```python
from build123d import *

# Parameters (mm, degrees)
BOSS_EXTRUDE1_DEPTH = 12.05
SKETCH2_R           = 1.25
BOSS_EXTRUDE2_DEPTH = 2.5
BOSS_EXTRUDE3_DEPTH = 4.4
SKETCH4_R           = 0.5
BOSS_EXTRUDE4_DEPTH = 3.7
CHAMFER1_SIZE       = 0.1


with BuildPart() as part:
    # Sketch1 → Boss-Extrude1 (new body, symmetric)
    with BuildSketch(Plane.XY):
        with BuildLine():
            Line((-5.6, -11.5), (5.6, -11.5))
            ThreePointArc((5.6, -11.5), (5.953553391, -11.353553391), (6.1, -11))
            Line((6.1, -11), (6.1, 11))
            ThreePointArc((6.1, 11), (5.953553391, 11.353553391), (5.6, 11.5))
            Line((5.6, 11.5), (-5.6, 11.5))
            ThreePointArc((-5.6, 11.5), (-5.953553391, 11.353553391), (-6.1, 11))
            Line((-6.1, 11), (-6.1, -11))
            ThreePointArc((-6.1, -11), (-5.953553391, -11.353553391), (-5.6, -11.5))
        make_face()
    extrude(amount=BOSS_EXTRUDE1_DEPTH, both=True)

    # Sketch2 → Boss-Extrude2 (add)
    with BuildSketch(Plane.XY.offset(-7.75)):
        with BuildLine():
            Line((6.1, 11), (6.1, 15.65))
            ThreePointArc((6.1, 15.65), (5.953553391, 16.003553391), (5.6, 16.15))
            Line((5.6, 16.15), (-5.6, 16.15))
            ThreePointArc((-5.6, 16.15), (-5.953553391, 16.003553391), (-6.1, 15.65))
            Line((-6.1, 15.65), (-6.1, 11))
            ThreePointArc((-6.1, 11), (-5.953553391, 11.353553391), (-5.6, 11.5))
            Line((-5.6, 11.5), (5.6, 11.5))
            ThreePointArc((5.6, 11.5), (5.953553391, 11.353553391), (6.1, 11))
        make_face()
        with Locations((0, 14.15)):
            Circle(SKETCH2_R, mode=Mode.SUBTRACT)
        with BuildLine():
            Line((5.6, -11.5), (-5.6, -11.5))
            ThreePointArc((-5.6, -11.5), (-5.953553391, -11.353553391), (-6.1, -11))
            Line((-6.1, -11), (-6.1, -15.65))
            ThreePointArc((-6.1, -15.65), (-5.953553391, -16.003553391), (-5.6, -16.15))
            Line((-5.6, -16.15), (5.6, -16.15))
            ThreePointArc((5.6, -16.15), (5.953553391, -16.003553391), (6.1, -15.65))
            Line((6.1, -15.65), (6.1, -11))
            ThreePointArc((6.1, -11), (5.953553391, -11.353553391), (5.6, -11.5))
        make_face()
        with Locations((0, -14.15)):
            Circle(SKETCH2_R, mode=Mode.SUBTRACT)
    extrude(amount=BOSS_EXTRUDE2_DEPTH)

    # Sketch3 → Boss-Extrude3 (add)
    with BuildSketch(Plane(origin=(0, 0, -12.05), x_dir=(-1, 0, 0), z_dir=(0, 0, -1))):
        with BuildLine():
            Line((-2.5, -1.6), (-2.5, -0.164171097))
            ThreePointArc((-2.5, -0.164171097), (0, 11.5), (2.5, -0.164171097))
            Line((2.5, -0.164171097), (2.5, -1.6))
            ThreePointArc((2.5, -1.6), (0, -4.1), (-2.5, -1.6))
        make_face()
    extrude(amount=BOSS_EXTRUDE3_DEPTH)

    # Sketch4 → Boss-Extrude4 (add)
    with BuildSketch(Plane(origin=(0, 0, -16.45), x_dir=(-1, 0, 0), z_dir=(0, 0, -1))):
        with Locations((0, 5.4)):
            Circle(SKETCH4_R)
    extrude(amount=BOSS_EXTRUDE4_DEPTH)

    # Chamfer1
    chamfer1_edges = [part.edges().sort_by_distance(p)[0] for p in [
        (0.5, 5.4, -20.15),
    ]]
    chamfer(chamfer1_edges, length=CHAMFER1_SIZE)


solid = part.part
```
Could you check a few things on this model? Use its own coordinates, in mm. A direction names the side the tool comes from. Coordinates: 2 decimals unless noted, no trailing zeros. Write each loop counter-clockwise with the first axis right and the second up, starting at its lowest first coordinate (ties: lowest second). Pieces come first, ordered by that corner, then holes. Notation, with made-up numbers: (36, -22.5) -> (87, -22.5) arc R19 cw to (87, -10.5) -> close; hole circle Ø11 at (-6, 61). An arc over 180 degrees is marked (long way). Return JSON: item names as keys, results as strings.
(1) Imagine slicing it at B-B, the plane z = -10. Please give me the cut outline in (x, y), then the cut area to 3 significant figures.
Numbers:
{"outline": "(-6.1, -11) arc R0.5 ccw to (-5.6, -11.5) -> (5.6, -11.5) arc R0.5 ccw to (6.1, -11) -> (6.1, 11) arc R0.5 ccw to (5.6, 11.5) -> (-5.6, 11.5) arc R0.5 ccw to (-6.1, 11) -> close", "area": "280 mm2"}
(2) Which directions (+Z, -Z, +X, -X, +Y, -Y) give clear straight access to the entire face, cutting with the end or side of a thin tool? Please do faces 1 (the flat face through (0, 11.5, 4)), 2 (the cylindrical face through (-0.1, -4.1, -14.2)), 3 (the flat face through (0, -11.5, -10)).
Numbers:
{"face 1": "+Z, +X, -X, +Y", "face 2": "-Z, -Y", "face 3": "-Z, +X, -X, -Y"}
(3) Imagine slicing it at A-A, the plane y = 14.15. Please give me the cut outline in (x, z), then the cut area to 4 significant figures.
Numbers:
{"outline": "(-6.1, -7.75) -> (-1.25, -7.75) -> (-1.25, -5.25) -> (-6.1, -5.25) -> close; (1.25, -7.75) -> (6.1, -7.75) -> (6.1, -5.25) -> (1.25, -5.25) -> close", "area": "24.25 mm2"}
(4) I need wall thicknesses on L1, parallel to Y at x = 0, z = -6.7; L2, parallel to Y at x = -5, z = -5; L3, parallel to Z at x = -5, y = 8.5. Which ranges of each line are inside material? Lowest first, please.
Numbers:
{"L1": "y = -16.15 to -15.4, -12.9 to 12.9, 15.4 to 16.15", "L2": "y = -11.5 to 11.5", "L3": "z = -16.45 to 12.05"}
(5) I'm going to push flat-ended pins straight in: pin 1 (1.1 mm diameter, centred on y = -0.5, z = -14, fed in from -X); pin 2 (1.5 mm diameter, centred on x = -2.5, y = 12.5, fed in from +Z); pin 3 (5 mm diameter, centred on x = -4.5, z = 6, fed in from -Y). Where does each tip first touch, or does it pass through?
Numbers:
{"pin 1": "stops at x = -2.93", "pin 2": "stops at z = -5.25", "pin 3": "stops at y = -11.5"}
(6) Imagine slicing it at D-D, the plane x = -4.25. Please give me the cut outline in (y, z), then the cut area to 3 significant figures.
Numbers:
{"outline": "(-16.15, -7.75) -> (-11.5, -7.75) -> (-11.5, -12.05) -> (1.02, -12.05) -> (1.02, -16.45) -> (9.78, -16.45) -> (9.78, -12.05) -> (11.5, -12.05) -> (11.5, -7.75) -> (16.15, -7.75) -> (16.15, -5.25) -> (11.5, -5.25) -> (11.5, 12.05) -> (-11.5, 12.05) -> (-11.5, -5.25) -> (-16.15, -5.25) -> close", "area": "616 mm2"}
(7) Imagine slicing it at C-C, the plane y = -2. Please give me the cut outline in (x, z).
Numbers:
{"outline": "(-6.1, -12.05) -> (-2.47, -12.05) -> (-2.47, -16.45) -> (2.47, -16.45) -> (2.47, -12.05) -> (6.1, -12.05) -> (6.1, 12.05) -> (-6.1, 12.05) -> close"}
